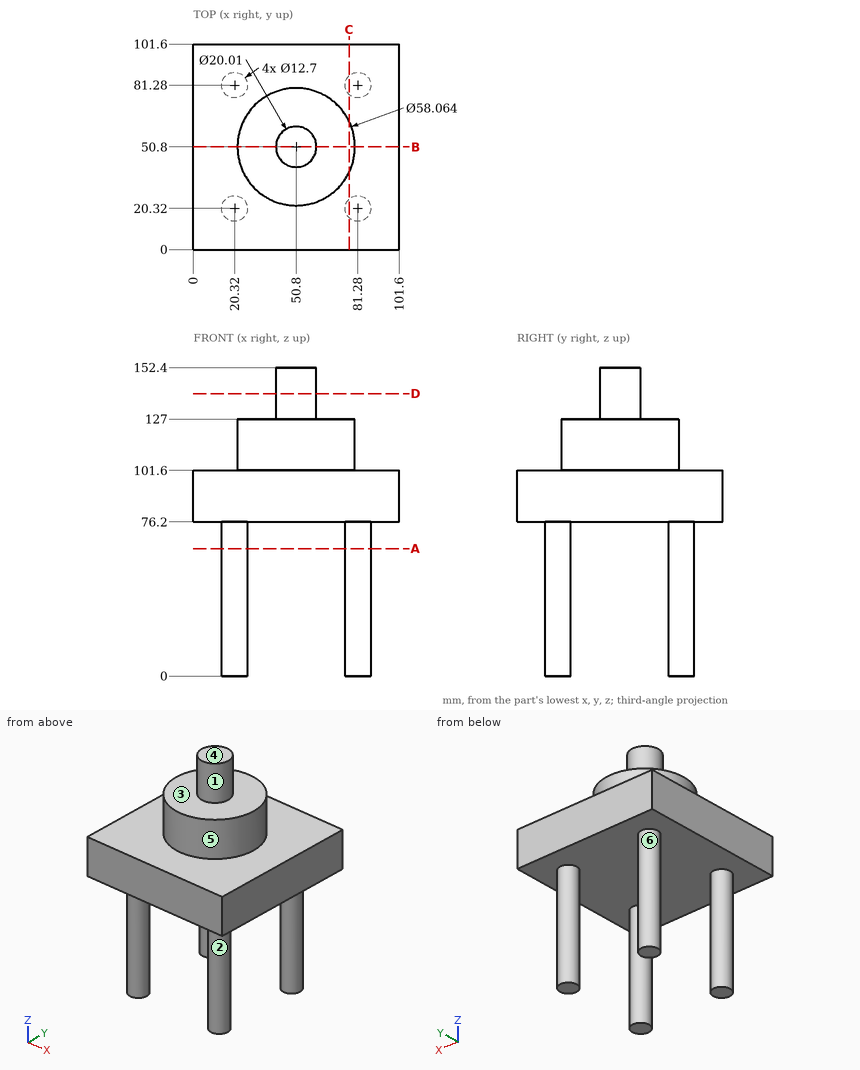
Drawing for the job (mm, zero at the part's lowest x, y, z). A direction names the side the tool comes from. Give positions to 0.01 mm unless a question says otherwise; leave off trailing zeros. Loops run counter-clockwise (first coordinate to the right, second up) from the corner with the lowest first, then second, coordinate; pieces in that order, holes last. Notation, with made-up numbers: (8, 64) - (43, 64) arc R21 cw to (43, 89) - close; hole circle Ø7 at (9, -6). An arc over 180 degrees is marked (long way). Write item = value, one per line. Start each with the question number.
1) Band-saw the part on A-A on z = 63. Give the cut face in (x, y), plus the area to 3 significant figures.
2) Drop flat-ended pins along their axis: pin 1 Ø3 at (x, y) = (47.5, 55.5) entering from -Z; pin 2 Ø5 at (x, y) = (79.5, 71) entering from +Z; pin 3 Ø12 at (x, y) = (33.5, 73) entering from +Z; pin 4 Ø12 at (x, y) = (90.5, 76) entering from -Z. Give the stop position or say it passes through.
3) Band-saw the part on B-B on y = 50.8. Give the cut face in (x, z) (1 decimal).
4) Probe probe 1 along Z at (x, y) = (5, 12); probe 2 along Y at (x, z) = (23, 21); probe 3 along Z at (x, y) = (77, 53). List the from-to ranges inside material, lowest first. Write a range as from..to.
5) Pull direction Y, two halves, no side cores. Call the marked faces 1, 2 and 3: +Y half, -Y half, draft (parallel to the pull), parting line (faces both ways), or undercut.
6) Band-saw the part on D-D on z = 139.5. Give the cut face in (x, y) (1 decimal).
7) Band-saw the part on C-C on x = 77. Give the cut face in (y, z), plus the area to 3 significant figures.
8) Tool access for the marked faces 4, 5 and 6: list every direction of +Z, -Z, +X, -X, +Y, -Y with a clear straight run to the whole face (end or side of a thin tool).
Final values:
q1.outline = circle Ø12.7 at (20.32, 20.32); circle Ø12.7 at (20.32, 81.28); circle Ø12.7 at (81.28, 20.32); circle Ø12.7 at (81.28, 81.28)
q1.area = 507 mm²
q2.pin_1 = 76.2
q2.pin_2 = 101.6
q2.pin_3 = 127
q2.pin_4 = 0
q3.outline = (0, 76.2) - (101.6, 76.2) - (101.6, 101.6) - (79.8, 101.6) - (79.8, 127) - (60.8, 127) - (60.8, 152.4) - (40.8, 152.4) - (40.8, 127) - (21.8, 127) - (21.8, 101.6) - (0, 101.6) - close
q4.probe_1 = 76.2..101.6
q4.probe_2 = 14.56..26.08, 75.52..87.04
q4.probe_3 = 76.2..127
q5.face_1 = parting line
q5.face_2 = undercut
q5.face_3 = draft
q6.outline = circle Ø20 at (50.8, 50.8)
q7.outline = (0, 76.2) - (15.63, 76.2) - (15.63, 0) - (25.01, 0) - (25.01, 76.2) - (76.59, 76.2) - (76.59, 0) - (85.97, 0) - (85.97, 76.2) - (101.6, 76.2) - (101.6, 101.6) - (63.31, 101.6) - (63.31, 127) - (38.29, 127) - (38.29, 101.6) - (0, 101.6) - close
q7.area = 4,650 mm²
q8.face_4 = +Z, +X, -X, +Y, -Y
q8.face_5 = +Z
q8.face_6 = -Z
